Read the model definition and answer for the solid it produces. Units are mm, in the model's axes. A direction names the side the tool comes from. Coordinates: 2 decimals unless noted, no trailing zeros. Loops run counter-clockwise (first coordinate to the right, second up) from the corner with the lowest first, then second, coordinate; pieces in that order, holes last. Notation, with made-up numbers: (67, -22.5) -> (122, -22.5) arc R18 cw to (122, 8.5) -> close; hole circle Ø4 at (-5.5, 31.25). An arc over 180 degrees is marked (long way). Answer in a Markdown table with one row per item.
Autodesk Inventor part; units mm, degrees
ref_plane "YZ Plane" through (0, 0, 0) normal (1, 0, 0) x (0, 1, 0)
ref_plane "XZ Plane" through (0, 0, 0) normal (0, 1, 0) x (-1, 0, 0)
ref_plane "XY Plane" through (0, 0, 0) normal (0, 0, 1) x (1, 0, 0)
sketch "Boceto1" plane through (0, 0, 0) normal (0, 1, 0) x (-1, 0, 0)
  circle A0 centre (0, 0) radius 8
  dimension "d0" = 16
extrude "Extrusión1" add sketch "Boceto1" along normal blind 15
sketch "Boceto5" plane through (0, 0, 0) normal (1, 0, 0) x (0, 1, 0)
  line L0 (15, -8) -> (15, 8)
  line L1 (15, -8) -> (24.831, -9.831)
  arc A0 (24.831, -9.831) -> (24.831, 9.831) centre (26.6619, 0) ccw
  line L2 (24.831, 9.831) -> (15, 8)
  point P0 (0, 0)
  point P1 (15, 0)
  dimension "d18" = 10
  dimension "d27" = 10
extrude "Extrusión5" add sketch "Boceto5" along normal mid plane 4
sketch "Boceto6" plane through (-2, 0, 0) normal (-1, 0, 0) x (0, 0, 1)
  arc A0 (9.831, 24.831) -> (-9.831, 24.831) centre (0, 26.6619) ccw
  circle A1 centre (0, 26.6619) radius 3
  point P0 (0, 0)
  dimension "d28" = 6
extrude "Extrusión6" cut sketch "Boceto6" against normal blind 4
sketch "Boceto7" plane through (0, 0, 0) normal (0, -1, 0) x (1, 0, 0)
  circle A0 centre (0, 0) radius 2.5
  dimension "d24" = 5
extrude "Extrusión7" cut sketch "Boceto7" against normal blind 14
properties part number "shocks_holder" material "Goma"
1. A tool of negligible diameter and unlimited length cuts with its end or side. For faces 5 (the flat face through (-4, 15, 0)), 6 (the flat face through (2, 0, -2)), 7 (the cylindrical face through (1.73, 7.4, 7.81)), 8 (the flat face through (-0.028, 19.847, -8.903)), 9 (the flat face through (4, 15, 0)), from which of +Z, -Z, +X, -X, +Y, -Y can it reach the whole face along a straight path? Write none if from no direction.
A:
| item | result |
|---|---|
| face 5 | +Z, -Z, -X, +Y |
| face 6 | +Z, -Z, +X, -X, -Y |
| face 7 | -Y |
| face 8 | -Z, +X, -X, -Y |
| face 9 | +Z, -Z, +X, +Y |
2. A cutting plane is placed at A-A on y = 26. Give the vertices of the cut face in (x, z).
A:
| item | result |
|---|---|
| outline | (-2, -9.98) -> (2, -9.98) -> (2, -2.93) -> (-2, -2.93) -> close; (-2, 2.93) -> (2, 2.93) -> (2, 9.98) -> (-2, 9.98) -> close |
3. A cutting plane is placed at B-B on z = 0. Give the vertices of the cut face in (x, y).
A:
| item | result |
|---|---|
| outline | (-8, 0) -> (-2.5, 0) -> (-2.5, 14) -> (2.5, 14) -> (2.5, 0) -> (8, 0) -> (8, 15) -> (2, 15) -> (2, 23.66) -> (-2, 23.66) -> (-2, 15) -> (-8, 15) -> close; (-2, 29.66) -> (2, 29.66) -> (2, 36.66) -> (-2, 36.66) -> close |
4. A cutting plane is placed at D-D on z = 5.5. Give the vertices of the cut face in (x, y), and give its area (3 significant figures).
A:
| item | result |
|---|---|
| outline | (-5.81, 0) -> (5.81, 0) -> (5.81, 15) -> (2, 15) -> (2, 35.01) -> (-2, 35.01) -> (-2, 15) -> (-5.81, 15) -> close |
| area | 254 mm2 |
5. The mould has two halves that part along X. Classify faces 1 (the flat face through (0, 14, 0)), 2 (the flat face through (-0.028, 19.984, 8.928)), 3 (the flat face through (-2, 23, 0)), 4 (the flat face through (2, 23, 0)): pulls with the +X half, pulls with the -X half, needs draft (parallel to the pull), parting line crosses it, or undercut.
A:
| item | result |
|---|---|
| face 1 | undercut |
| face 2 | needs draft |
| face 3 | pulls with the -X half |
| face 4 | pulls with the +X half |
6. Find the intervals of material crossed by probe 1 along Y at (x, z) = (-1, 0); probe 2 along X at (y, z) = (25.5, -3); probe 3 along Z at (x, y) = (0, 7.5), in increasing order.
A:
| item | result |
|---|---|
| probe 1 | y = 14 to 23.66, 29.66 to 36.66 |
| probe 2 | x = -2 to 2 |
| probe 3 | z = -8 to -2.5, 2.5 to 8 |
7. A cutting plane is placed at C-C on y = 3. Give the vertices of the cut face in (x, z).
A:
| item | result |
|---|---|
| outline | circle Ø16 at (0, 0); hole circle Ø5 at (0, 0) |
8. Given pin 1 Ø6 at (y, z) = (24, -2.5) entering from -X; pin 2 Ø10 at (y, z) = (30.5, 2.5) entering from +X; pin 3 Ø1 at (x, z) = (-3.5, -2.5) entering from +Y, each flat-ended and moving along its own axis, determine where each tip first touches the part or whether it passes through.
A:
| item | result |
|---|---|
| pin 1 | stops at x = -2 |
| pin 2 | stops at x = 2 |
| pin 3 | stops at y = 15 |
